from build123d import *

# Parameters (mm, degrees)
SKETCH1_R           = 7.5
SKETCH1_R_2         = 5.15
BOSS_EXTRUDE1_DEPTH = 5
SKETCH1_3_R         = 5.15
BOSS_EXTRUDE2_DEPTH = 15.7
BOSS_EXTRUDE3_DEPTH = 4
SKETCH3_R           = 1.625
CUT_EXTRUDE1_DEPTH  = 37
SKETCH4_R           = 3.5
CUT_EXTRUDE2_DEPTH  = 10.7
BOSS_EXTRUDE4_START = 3.5
SKETCH5_R           = 7.5
SKETCH5_R_2         = 3.5
BOSS_EXTRUDE4_DEPTH = 3.5
BOSS_EXTRUDE5_START = 4
SKETCH6_R           = 15
SKETCH6_R_2         = 3.5
SKETCH6_R_3         = 1.375
BOSS_EXTRUDE5_DEPTH = 4
SKETCH7_R           = 3
CUT_EXTRUDE3_DEPTH  = 1
CUT_EXTRUDE4_START  = -12.5
SKETCH8_R           = 7.5
SKETCH8_R_2         = 7.45
CUT_EXTRUDE4_DEPTH  = 12.5


with BuildPart() as part:
    # Sketch1 → Boss-Extrude1 (new body)
    # profile 1 of 2: a face of its own
    with BuildSketch(Plane(origin=(0, 0, 0), x_dir=(1, 0, 0), z_dir=(0, 1, 0))):
        with Locations(Location((0, 0, 0), (0, 0, 270))):
            Circle(SKETCH1_R)
        Circle(SKETCH1_R_2, mode=Mode.SUBTRACT)
    # profile 2 of 2: a face of its own
    with BuildSketch(Plane(origin=(0, 0, 0), x_dir=(1, 0, 0), z_dir=(0, 1, 0))):
        Circle(SKETCH1_R_2)
    extrude(amount=BOSS_EXTRUDE1_DEPTH)

    # Sketch1_3 → Boss-Extrude2 (add)
    with BuildSketch(Plane(origin=(0, 0, 0), x_dir=(1, 0, 0), z_dir=(0, 1, 0))):
        with Locations(Location((0, 0, 0), (0, 0, 270))):
            Circle(SKETCH1_3_R)
    extrude(amount=BOSS_EXTRUDE2_DEPTH)

    # Sketch2 → Boss-Extrude3 (add)
    with BuildSketch(Plane(origin=(0, 5, 0), x_dir=(1, 0, 0), z_dir=(0, 1, 0))):
        with BuildLine():
            ThreePointArc((7.5, 0), (5.303300859, 5.303300859), (0, 7.5))
            Line((0, 7.5), (0, 5.15))
            ThreePointArc((0, 5.15), (3.641599923, 3.641599923), (5.15, 0))
            ThreePointArc((5.15, 0), (3.641599923, -3.641599923), (0, -5.15))
            Line((0, -5.15), (0, -7.5))
            ThreePointArc((0, -7.5), (5.303300859, -5.303300859), (7.5, 0))
        make_face()
    extrude(amount=BOSS_EXTRUDE3_DEPTH)

    # Sketch3 → Cut-Extrude1 (cut)
    with BuildSketch(Plane.XZ):
        with Locations(Location((0, 0, 0), (0, 0, 270))):
            Circle(SKETCH3_R)
    extrude(amount=-CUT_EXTRUDE1_DEPTH, mode=Mode.SUBTRACT)

    # Sketch4 → Cut-Extrude2 (cut)
    with BuildSketch(Plane.XZ):
        with Locations(Location((0, 0, 0), (0, 0, 270))):
            Circle(SKETCH4_R)
    extrude(amount=-CUT_EXTRUDE2_DEPTH, mode=Mode.SUBTRACT)

    # Sketch5 → Boss-Extrude4 (add)
    with BuildSketch(Plane.XZ.offset(BOSS_EXTRUDE4_START)):
        with Locations(Location((0, 0, 0), (0, 0, 270))):
            Circle(SKETCH5_R)
        with Locations(Location((0, 0, 0), (0, 0, 270))):
            Circle(SKETCH5_R_2, mode=Mode.SUBTRACT)
    extrude(amount=-BOSS_EXTRUDE4_DEPTH)

    # Sketch6 → Boss-Extrude5 (add)
    with BuildSketch(Plane.XZ.offset(3.5).offset(BOSS_EXTRUDE5_START)):
        with Locations(Location((0, 0, 0), (0, 0, 270))):
            Circle(SKETCH6_R)
        with Locations(Location((0, 0, 0), (0, 0, 270))):
            Circle(SKETCH6_R_2, mode=Mode.SUBTRACT)
        with Locations(Location((-11, 0, 0), (0, 0, 270))):
            Circle(SKETCH6_R_3, mode=Mode.SUBTRACT)
        with Locations(Location((-7.778174593, 7.778174593, 0), (0, 0, 270))):
            Circle(SKETCH6_R_3, mode=Mode.SUBTRACT)
        with Locations(Location((0, 11, 0), (0, 0, 270))):
            Circle(SKETCH6_R_3, mode=Mode.SUBTRACT)
        with Locations(Location((7.778174593, 7.778174593, 0), (0, 0, 270))):
            Circle(SKETCH6_R_3, mode=Mode.SUBTRACT)
        with Locations(Location((11, 0, 0), (0, 0, 270))):
            Circle(SKETCH6_R_3, mode=Mode.SUBTRACT)
        with Locations(Location((7.778174593, -7.778174593, 0), (0, 0, 270))):
            Circle(SKETCH6_R_3, mode=Mode.SUBTRACT)
        with Locations(Location((0, -11, 0), (0, 0, 270))):
            Circle(SKETCH6_R_3, mode=Mode.SUBTRACT)
        with Locations(Location((-7.778174593, -7.778174593, 0), (0, 0, 270))):
            Circle(SKETCH6_R_3, mode=Mode.SUBTRACT)
    extrude(amount=-BOSS_EXTRUDE5_DEPTH)

    # Sketch7 → Cut-Extrude3 (cut)
    with BuildSketch(Plane(origin=(0, -3.5, 0), x_dir=(1, 0, 0), z_dir=(0, 1, 0))):
        with Locations(Location((-11, 0, 0), (0, 0, 270))):
            Circle(SKETCH7_R)
        with Locations(Location((-7.778174593, 7.778174593, 0), (0, 0, 270))):
            Circle(SKETCH7_R)
        with Locations(Location((0, 11, 0), (0, 0, 270))):
            Circle(SKETCH7_R)
        with Locations(Location((7.778174593, 7.778174593, 0), (0, 0, 270))):
            Circle(SKETCH7_R)
        with Locations(Location((11, 0, 0), (0, 0, 270))):
            Circle(SKETCH7_R)
        with Locations(Location((7.778174593, -7.778174593, 0), (0, 0, 270))):
            Circle(SKETCH7_R)
        with Locations(Location((0, -11, 0), (0, 0, 270))):
            Circle(SKETCH7_R)
        with Locations(Location((-7.778174593, -7.778174593, 0), (0, 0, 270))):
            Circle(SKETCH7_R)
    extrude(amount=-CUT_EXTRUDE3_DEPTH, mode=Mode.SUBTRACT)

    # Sketch8 → Cut-Extrude4 (cut)
    with BuildSketch(Plane(origin=(0, 9, 0), x_dir=(1, 0, 0), z_dir=(0, 1, 0)).offset(CUT_EXTRUDE4_START)):
        Circle(SKETCH8_R)
        with Locations(Location((0, 0, 0), (0, 0, 270))):
            Circle(SKETCH8_R_2, mode=Mode.SUBTRACT)
    extrude(amount=CUT_EXTRUDE4_DEPTH, mode=Mode.SUBTRACT)


solid = part.part
Model file for the job. Use its own axes, mm. A direction names the side the tool comes from. Give positions to 0.01 mm unless a question says otherwise; leave off trailing zeros. Order: outer loops, then holes, each group sorted by start corner. A loop starts at its lowest first (then second) coordinate and runs counter-clockwise, first axis right, second up. Notation, with made-up numbers: (72, 82) - (97, 82) arc R32 ccw to (97, 109) - close; hole circle Ø7 at (74, 30.5). An arc over 180 degrees is marked (long way). Return JSON: item names as keys, results as strings.
1) Cut at C-C, the plane x = -8.5. Give the cut face in (y, z), plus the area to 3 significant figures.
Geometry says:
{"outline": "(-7.5, -12.36) - (-3.5, -12.36) - (-3.5, -10.69) - (-4.5, -10.69) - (-4.5, -8.95) - (-7.5, -8.95) - close; (-7.5, -6.61) - (-4.5, -6.61) - (-4.5, -4.87) - (-3.5, -4.87) - (-3.5, -1.66) - (-4.5, -1.66) - (-4.5, 1.66) - (-3.5, 1.66) - (-3.5, 4.87) - (-4.5, 4.87) - (-4.5, 6.61) - (-7.5, 6.61) - close; (-7.5, 8.95) - (-4.5, 8.95) - (-4.5, 10.69) - (-3.5, 10.69) - (-3.5, 12.36) - (-7.5, 12.36) - close", "area": "69.9 mm²"}
2) Cut at B-B, the plane y = 5.5. Give the cut face in (x, z), plus the area to 3 significant figures.
Geometry says:
{"outline": "(0, -7.45) arc R7.45 ccw to (0, 7.45) - (0, 5.15) arc R5.15 ccw to (0, -5.15) - close; hole circle Ø7 at (0, 0)", "area": "90.4 mm²"}
3) Probe line 1 (X direction, y = -5.7, z = 0) (3 decimals); line 2 (Y direction, x = -3, z = 7.5); line 3 (Y direction, x = 5.25, z = -0.75). List the from-to ranges inside material, lowest first. Write a range as from..to.
Geometry says:
{"line 1": "-15..-12.375, -9.625..-3.5, 3.5..9.625, 12.375..15", "line 2": "-7.5..-3.5", "line 3": "-7.5..9"}
4) Flat gauge pins, fed straight in: P1, Ø12, axis at y = 13.5, z = -0.5, coming from the +X side; P2, Ø8, axis at y = 2, z = -7, coming from the -X side; P3, Ø6.5, axis at x = 8, z = 6.5, coming from the +Y side; P4, Ø2, axis at x = 7.78, z = 7.78, coming from the +Y side. Where does each tip first touch, or does it go through?
Geometry says:
{"P1": "x = 7.45", "P2": "x = -6.82", "P3": "y = 9", "P4": "through"}
5) Pull direction Z, two halves, no side cores. Call faces 1 (the flat face through (5.3, 9, -0.1)), 2 (the cylindrical face through (-4.569, 11.464, 2.376)), 3 (the cylindrical face through (-9, -6.02, -8.41)): pulls with the +Z half, pulls with the -Z half, needs draft (parallel to the pull), parting line crosses it, or undercut.
Geometry says:
{"face 1": "needs draft", "face 2": "parting line crosses it", "face 3": "undercut"}
6) Cut at A-A, the plane z = -11.5. Give the cut face in (x, y), plus the area to 3 significant figures.
Geometry says:
{"outline": "(-9.63, -7.5) - (-1.28, -7.5) - (-1.28, -4.5) - (-2.96, -4.5) - (-2.96, -3.5) - (-9.63, -3.5) - close; (1.28, -7.5) - (9.63, -7.5) - (9.63, -3.5) - (2.96, -3.5) - (2.96, -4.5) - (1.28, -4.5) - close", "area": "63.4 mm²"}
7) Cut at D-D, the plane z = 0. Count the separate pieces of the cut face and the enclosed holes in it, plus the area to 3 significant figures.
Geometry says:
{"separate pieces": "4", "enclosed holes": "0", "area": "194 mm²"}
8) 3-axis set-ups, long thin cutter, end or side, ignore diameter. For faces 4 (the flat face through (4, -7.5, 0)), 5 (the flat face through (-5.3, 5, -0.1)), 6 (the flat face through (0, 7, 6)), 7 (the cylindrical face through (-5.25, -3.99, 9.39)), 8 (the cylindrical face through (-3.417, 1.473, 0.759)): which of +Z, -Z, +X, -X, +Y, -Y reach the whole face in a straight line?
Geometry says:
{"face 4": "+Z, -Z, +X, -X, -Y", "face 5": "-X, +Y", "face 6": "+Z, -X, +Y", "face 7": "+Y", "face 8": "-Y"}
